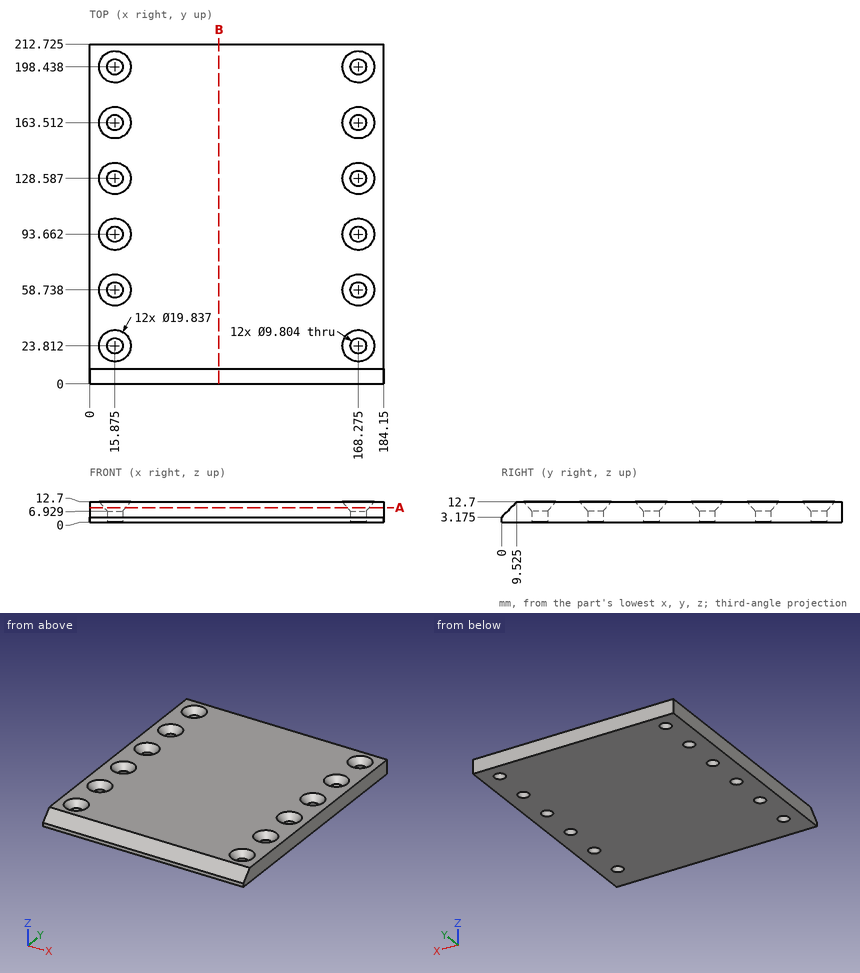
Geometry check sheet. Reference: drawing and pictorial views, mm from the part's lowest x, y, z. Give positions to 0.01 mm unless a question says otherwise; leave off trailing zeros. Loops run counter-clockwise (first coordinate to the right, second up) from the corner with the lowest first, then second, coordinate; pieces in that order, holes last.
1. Go/stop test with flat-tipped pins: pin 1 Ø9 at (x, y) = (168.28, 58.74) entering from -Z; pin 2 Ø11.5 at (x, y) = (15.88, 163.51) entering from +Z; pin 3 Ø15.5 at (x, y) = (15.88, 23.81) entering from +Z; pin 4 Ø1 at (x, z) = (122, 7) entering from -Y (1 decimal). Record where each tip stops, or that it passes through.
2. Thickness scan on line 1 (X direction, y = 27, z = 11); line 2 (X direction, y = 62.5, z = 11); line 3 (Y direction, x = 120, z = 8.75) (1 decimal). Record the ranges inside material, lowest first.
3. Section check A-A, the plane z = 9. Count the separate pieces of the cut face and the enclosed holes in it, then the cut area to 3 significant figures.
4. Section check B-B, the plane x = 81. Enter the section's corners in (y, z) (1 decimal), then the cut area to 3 significant figures.
Geometry says:
1. pin 1: passes through
1. pin 2: stops at z = 7.91
1. pin 3: stops at z = 10.21
1. pin 4: stops at y = 3.3
2. line 1: x = 0 to 8.06, 23.69 to 160.46, 176.09 to 184.15
2. line 2: x = 0 to 8.32, 23.43 to 160.72, 175.83 to 184.15
2. line 3: y = 5.6 to 212.7
3. separate pieces: 1
3. enclosed holes: 12
3. area: 36,400 mm2
4. outline: (0, 0) - (212.7, 0) - (212.7, 12.7) - (9.5, 12.7) - (0, 3.2) - close
4. area: 2,660 mm2
